Read the model definition and answer for the solid it produces. Units are mm, in the model's axes. A direction names the side the tool comes from. Coordinates: 2 decimals unless noted, no trailing zeros. Write each loop counter-clockwise with the first axis right and the second up, starting at its lowest first coordinate (ties: lowest second). Pieces come first, ordered by that corner, then holes. Notation, with made-up numbers: (59.25, 83) - (114.25, 83) arc R18 cw to (114.25, 99) - close; hole circle Ø6 at (41, 74.5). An arc over 180 degrees is marked (long way). Use a Markdown table: item, result.
from build123d import *

# Parameters (mm, degrees)
SKETCH1_R           = 25
BOSS_EXTRUDE1_DEPTH = 80
SKETCH2_R           = 17.5
BOSS_EXTRUDE2_DEPTH = 16
SKETCH3_R           = 10
CUT_EXTRUDE1_DEPTH  = 144
BOSS_EXTRUDE3_DEPTH = 40
SKETCH5_W           = 30
SKETCH5_H           = 40
SKETCH5_W_2         = 20
SKETCH5_W_3         = 10
BOSS_EXTRUDE4_DEPTH = 10
SKETCH6_W           = 10
SKETCH6_H           = 40
BOSS_EXTRUDE5_DEPTH = 35
CUT_EXTRUDE2_DEPTH  = 35


with BuildPart() as part:
    # Sketch1 → Boss-Extrude1 (new body)
    with BuildSketch(Plane(origin=(0, 0, 0), x_dir=(1, 0, 0), z_dir=(0, 1, 0))):
        with Locations(Location((0, 0, 0), (0, 0, 270))):
            Circle(SKETCH1_R)
    extrude(amount=BOSS_EXTRUDE1_DEPTH)

    # Sketch2 → Boss-Extrude2 (add)
    with BuildSketch(Plane(origin=(0, 80, 0), x_dir=(1, 0, 0), z_dir=(0, 1, 0))):
        with Locations(Location((0, 0, 0), (0, 0, 270))):
            Circle(SKETCH2_R)
    extrude(amount=BOSS_EXTRUDE2_DEPTH)

    # Sketch3 → Cut-Extrude1 (cut)
    with BuildSketch(Plane(origin=(0, 96, 0), x_dir=(1, 0, 0), z_dir=(0, 1, 0))):
        with Locations(Location((0, 0, 0), (0, 0, 270))):
            Circle(SKETCH3_R)
    extrude(amount=-CUT_EXTRUDE1_DEPTH, mode=Mode.SUBTRACT)

    # Sketch4 → Boss-Extrude3 (add)
    with BuildSketch(Plane(origin=(0, 50, 0), x_dir=(1, 0, 0), z_dir=(0, 1, 0))):
        Polygon((0, -35), (0, 0), (-25, 0), (-25, -65), (-15, -65), (-15, -35), align=None)
        Polygon((25, 0), (0, 0), (0, -35), (15, -35), (15, -65), (25, -65), align=None)
    extrude(amount=-BOSS_EXTRUDE3_DEPTH)

    # Sketch5 → Boss-Extrude4 (add)
    with BuildSketch(Plane.XY.offset(65)):
        with Locations((-30, 30)):
            Rectangle(SKETCH5_W, SKETCH5_H)
        with Locations((35, 30)):
            Rectangle(SKETCH5_W_2, SKETCH5_H)
        with Locations((20, 30)):
            Rectangle(SKETCH5_W_3, SKETCH5_H)
    extrude(amount=BOSS_EXTRUDE4_DEPTH)

    # Sketch6 → Boss-Extrude5 (add)
    with BuildSketch(Plane.XY.offset(75)):
        with Locations((-40, 30)):
            Rectangle(SKETCH6_W, SKETCH6_H)
    boss_extrude5 = extrude(amount=BOSS_EXTRUDE5_DEPTH)

    # Sketch7 → Cut-Extrude2 (cut)
    with BuildSketch(Plane(origin=(-35, 0, 0), x_dir=(0, 0, -1), z_dir=(1, 0, 0))):
        with BuildLine():
            Line((-107.082039325, 50), (-110, 50))
            Line((-110, 50), (-110, 30))
            ThreePointArc((-110, 30), (-109.266668581, 40.10587075), (-107.082039325, 50))
        make_face()
        with BuildLine():
            ThreePointArc((-107.082039325, 10), (-109.266668581, 19.89412925), (-110, 30))
            Line((-110, 30), (-110, 10))
            Line((-110, 10), (-107.082039325, 10))
        make_face()
        with BuildLine():
            ThreePointArc((-81.5, 30), (-87.5, 36), (-93.5, 30))
            Line((-93.5, 30), (-87.5, 30))
            Line((-87.5, 30), (-81.5, 30))
        make_face()
        with BuildLine():
            Line((-87.5, 30), (-93.5, 30))
            ThreePointArc((-93.5, 30), (-87.5, 24), (-81.5, 30))
            Line((-81.5, 30), (-87.5, 30))
        make_face()
    cut_extrude2 = extrude(amount=-CUT_EXTRUDE2_DEPTH, mode=Mode.SUBTRACT)

    # Mirror1: Boss-Extrude5, Cut-Extrude2 across plane
    add(boss_extrude5.mirror(Plane(origin=(0, 0, 0), x_dir=(0, 0, 1), z_dir=(1, 0, 0))))
    add(cut_extrude2.mirror(Plane(origin=(0, 0, 0), x_dir=(0, 0, 1), z_dir=(1, 0, 0))), mode=Mode.SUBTRACT)


solid = part.part
(1) A cutting plane is placed at B-B, the plane z = -7.5. Write down the section's boundary in (x, y).
Report:
| item | result |
|---|---|
| outline | (-23.85, 0) - (-6.61, 0) - (-6.61, 96) - (-15.81, 96) - (-15.81, 80) - (-23.85, 80) - close; (6.61, 0) - (23.85, 0) - (23.85, 80) - (15.81, 80) - (15.81, 96) - (6.61, 96) - close |
(2) For faces 1 (the cylindrical face through (-10.648, 87.888, -13.887)), 2 (the flat face through (-25, 30, 32)), 3 (the flat face through (35, 30, 65)), determine the directions among +Z, -Z, +X, -X, +Y, -Y from which every point of the face is accessible in a straight line to the end or side of a thin tool.
Report:
| item | result |
|---|---|
| face 1 | +Y |
| face 2 | -Z, -X, +Y, -Y |
| face 3 | -Z, +X, +Y, -Y |
(3) Each of these flat-tipped pins is pushed along its axis until it touches: P1, Ø12, axis at y = 20.5, z = 51.5, coming from the -X side; P2, Ø22, axis at x = -33, y = 36, coming from the -Z side; P3, Ø12, axis at x = -12, y = 33.5, coming from the -Z side. Where does it stop, or does it pass through?
Report:
| item | result |
|---|---|
| P1 | stops at x = -25 |
| P2 | stops at z = -11.87 |
| P3 | stops at z = -24.27 |
(4) A cutting plane is placed at A-A, the plane x = 0. Write down the section's boundary in (y, z).
Report:
| item | result |
|---|---|
| outline | (0, -25) - (80, -25) - (80, -17.5) - (96, -17.5) - (96, -10) - (0, -10) - close; (0, 10) - (10, 10) - (10, 0) - (50, 0) - (50, 10) - (96, 10) - (96, 17.5) - (80, 17.5) - (80, 25) - (50, 25) - (50, 35) - (10, 35) - (10, 25) - (0, 25) - close |
(5) Straight lines are drawn through the part: L1, parallel to Y at x = 38.75, z = 87.5; L2, parallel to Z at x = -37.25, y = 30; L3, parallel to X at y = 55, z = 0. For each, find the intervals that lie inside material, in ascending order.
Report:
| item | result |
|---|---|
| L1 | y = 10 to 24, 36 to 50 |
| L2 | z = 65 to 81.5, 93.5 to 110 |
| L3 | x = -25 to -10, 10 to 25 |
(6) A cutting plane is placed at C-C, the plane x = 39. Write down the section's boundary in (y, z), and give its area (3 significant figures).
Report:
| item | result |
|---|---|
| outline | (10, 65) - (50, 65) - (50, 107.08) arc R70 ccw to (10, 107.08) - close; hole circle Ø12 at (30, 87.5) |
| area | 1,650 mm² |
(7) The mould has two halves that part along Z. Classify faces 4 (the flat face through (-15, 30, 55)), 5 (the cylindrical face through (1.099, 39.44, -24.976)), 6 (the flat face through (0, 30, 0)): pulls with the +Z half, pulls with the -Z half, needs draft (parallel to the pull), parting line crosses it, or undercut.
Report:
| item | result |
|---|---|
| face 4 | needs draft |
| face 5 | parting line crosses it |
| face 6 | undercut |
(8) A cutting plane is placed at D-D, the plane y = 44. Write down the section's boundary in (x, z).
Report:
| item | result |
|---|---|
| outline | (-45, 65) - (-25, 65) - (-25, 0) arc R25 ccw to (25, 0) - (25, 65) - (45, 65) - (45, 108.59) - (35, 108.59) - (35, 75) - (15, 75) - (15, 35) - (-15, 35) - (-15, 75) - (-35, 75) - (-35, 108.59) - (-45, 108.59) - close; hole (-10, 0) arc R10 ccw to (10, 0) - close |
